Input: part model. Units: mm. Frame: model coordinates. Round coordinates to 2 decimals unless told otherwise and drop trailing zeros. Loops run counter-clockwise (first coordinate to the right, second up) from the corner with the lowest first, then second, coordinate; pieces in that order, holes last. Notation, with made-up numbers: M -4.75,-5.5 L 22.25,-5.5 A12 cw 22.25,0.5 Z; hole C -11,61.25 d3. An arc over 180 degrees is marked long. Return JSON: item names as keys, results as strings. Group by question number.
1) Section C-C (z = 89). Output: boundary loops of the cut face in (x, y).
2) Section B-B (y = 64). Output: boundary loops of the cut face in (x, z), plus the area to 3 significant figures.
3) Contact query for flat-ended pins moving along their axis: P1, Ø10, axis at x = -17, y = 12.5, coming from the +Z side; P2, Ø3, axis at x = -14, z = 30, coming from the -Y side; P3, Ø1, axis at x = 20.5, z = 46, coming from the -Y side. Output: stop coordinate, or through.
4) Material intervals for line 1 (Z direction, x = 30, y = 30.5); line 2 (Y direction, x = 23.5, z = 35); line 3 (Y direction, x = 10, z = -19), sorted ascending. Write a range as from..to.
5) Section A-A (x = 30.5). Output: boundary loops of the cut face in (y, z).
from build123d import *

# Parameters (mm, degrees)
BOSS_EXTRUDE1_DEPTH = 38.1
FILLET1_R           = 1.27


with BuildPart() as part:
    # Sketch1 → Boss-Extrude1 (new, symmetric)
    with BuildSketch(Plane(origin=(0, 0, 0), x_dir=(0, 0, -1), z_dir=(1, 0, 0))):
        with BuildLine():
            Line((28.422826333, 0), (-28.422826333, 0))
            Line((-28.422826333, 0), (-127.802622568, 21.123827787))
            ThreePointArc((-127.802622568, 21.123827787), (-41.944172269, 26.690897226), (28.422826333, 76.2))
            Line((28.422826333, 76.2), (28.422826333, 0))
        make_face()
    extrude(amount=BOSS_EXTRUDE1_DEPTH, both=True)

    # Fillet1
    fillet1_edges = [part.edges().sort_by_distance(p)[0] for p in [
        (0, 76.2, -28.422826333),
    ]]
    fillet(fillet1_edges, radius=FILLET1_R)
    fillet1_2_edges = [part.edges().sort_by_distance(p)[0] for p in [
        (0, 21.123827787, 127.802622568),
    ]]
    fillet(fillet1_2_edges, radius=FILLET1_R)


solid = part.part
Returned:
{
 "1": {"outline": "M -38.1,12.88 L 38.1,12.88 L 38.1,17.76 L -38.1,17.76 Z"},
 "2": {"outline": "M -38.1,-28.42 L 38.1,-28.42 L 38.1,-17.39 L -38.1,-17.39 Z", "area": "841 mm^2"},
 "3": {"P1": "stops at z = 101.02", "P2": "stops at y = 0.02", "P3": "stops at y = 3.63"},
 "4": {"line 1": "z = -28.42..32.18", "line 2": "y = 1.4..29.32", "line 3": "y = 0..65.63"},
 "5": {"outline": "M 0,-28.42 L 72.69,-28.42 A1.27 ccw 73.51,-26.19 A158.88 cw 17.73,99.71 A1.27 ccw 15.22,100.01 L 0,28.42 Z"}
}
